Part model, mm, in its own coordinate system. Coordinates: 2 decimals unless noted, no trailing zeros. Write each loop counter-clockwise with the first axis right and the second up, starting at its lowest first coordinate (ties: lowest second). Pieces come first, ordered by that corner, then holes. Notation, with made-up numbers: (88.5, 65.5) - (98.5, 65.5) arc R21 ccw to (98.5, 75.5) - close; hole circle Ø4 at (-28.75, 12). An arc over 180 degrees is marked (long way). Use a Markdown table: item, result.
```python
from build123d import *

# Parameters (mm, degrees)
SKETCH1_R           = 7.95
BOSS_EXTRUDE1_DEPTH = 12.75
FILLET1_R           = 1.5
SKETCH2_R           = 6.45
CUT_EXTRUDE1_DEPTH  = 2
FILLET2_R           = 1.5


with BuildPart() as part:
    # Sketch1 → Boss-Extrude1 (new body)
    with BuildSketch(Plane(origin=(0, 0, 0), x_dir=(1, 0, 0), z_dir=(0, 1, 0))):
        with Locations(Location((0, 0, 0), (0, 0, 270))):
            Circle(SKETCH1_R)
    extrude(amount=BOSS_EXTRUDE1_DEPTH)

    # Fillet1
    fillet1_edges = [part.edges().sort_by_distance(p)[0] for p in [
        (0, 12.75, -7.95),
    ]]
    fillet(fillet1_edges, radius=FILLET1_R)

    # Sketch2 → Cut-Extrude1 (cut)
    with BuildSketch(Plane(origin=(0, 12.75, 0), x_dir=(1, 0, 0), z_dir=(0, 1, 0))):
        with Locations(Location((0, 0, 0), (0, 0, 270))):
            Circle(SKETCH2_R)
    extrude(amount=-CUT_EXTRUDE1_DEPTH, mode=Mode.SUBTRACT)

    # Fillet2
    fillet2_edges = [part.edges().sort_by_distance(p)[0] for p in [
        (0, 10.75, -6.45),
    ]]
    fillet(fillet2_edges, radius=FILLET2_R)


solid = part.part
```
Item 1: Drill centre lines: probe 1 along Y at (x, z) = (-2, 2.25); probe 2 along X at (y, z) = (1.25, -0.25); probe 3 along X at (y, z) = (12.5, 0). Where is each one in solid material? Low to high.
From the geometry:
| item | result |
|---|---|
| probe 1 | 0 to 10.75 |
| probe 2 | -7.95 to 7.95 |
| probe 3 | -7.28 to -6.45, 6.45 to 7.28 |
Item 2: Band-saw the part on B-B, the plane x = 0. Give the cut face in (y, z).
From the geometry:
| item | result |
|---|---|
| outline | (0, -7.95) - (11.25, -7.95) arc R1.5 ccw to (12.75, -6.45) - (12.25, -6.45) arc R1.5 cw to (10.75, -4.95) - (10.75, 4.95) arc R1.5 cw to (12.25, 6.45) - (12.75, 6.45) arc R1.5 ccw to (11.25, 7.95) - (0, 7.95) - close |
Item 3: Drop flat-ended pins along their axis: P1, Ø1, axis at y = 7, z = -1.5, coming from the -X side; P2, Ø5, axis at x = -1, z = -1, coming from the +Y side; P3, Ø8, axis at x = 1.5, z = -1, coming from the +Y side. Give the stop position or say it passes through.
From the geometry:
| item | result |
|---|---|
| P1 | x = -7.89 |
| P2 | y = 10.75 |
| P3 | y = 11.02 |
Item 4: Two-plate mould, pull along Z, no slides. Class faces 1 (the face through (0, 0, 0)), 2 (the face through (0, 10.75, 0)), 3 (the face through (-4.837, 5.546, -6.309)): pulls with the +Z half, pulls with the -Z half, needs draft (parallel to the pull), parting line crosses it, or undercut.
From the geometry:
| item | result |
|---|---|
| face 1 | needs draft |
| face 2 | undercut |
| face 3 | parting line crosses it |
Item 5: Band-saw the part on C-C, the plane y = 2.5. Give the cut face in (x, z), then the cut area to 3 significant figures.
From the geometry:
| item | result |
|---|---|
| outline | circle Ø15.9 at (0, 0) |
| area | 199 mm^2 |
Item 6: Band-saw the part on D-D, the plane y = 11. Give the cut face in (x, z).
From the geometry:
| item | result |
|---|---|
| outline | circle Ø15.9 at (0, 0); hole circle Ø11.56 at (0, 0) |
Item 7: Band-saw the part on A-A, the plane z = 0. Give the cut face in (x, y), then the cut area to 3 significant figures.
From the geometry:
| item | result |
|---|---|
| outline | (-7.95, 0) - (7.95, 0) - (7.95, 11.25) arc R1.5 ccw to (6.45, 12.75) - (6.45, 12.25) arc R1.5 cw to (4.95, 10.75) - (-4.95, 10.75) arc R1.5 cw to (-6.45, 12.25) - (-6.45, 12.75) arc R1.5 ccw to (-7.95, 11.25) - close |
| area | 177 mm^2 |
